For this review, use the dimensioned drawing (mm, ordinates from the lowest corner) and the shaded views. Round coordinates to 2 decimals unless told otherwise and drop trailing zeros. Write each loop counter-clockwise with the first axis right and the second up, starting at its lowest first coordinate (ties: lowest second). Pieces come first, ordered by that corner, then holes.
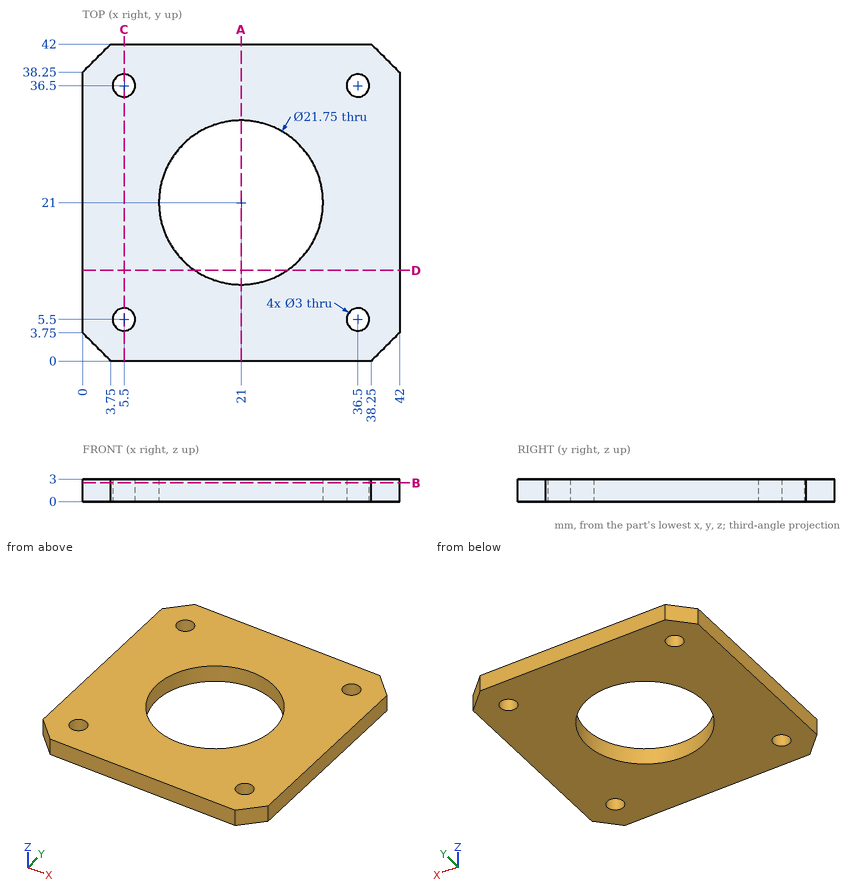
1) Add section B-B on z = 2.5. State the section outline as (x, y) points (3 decimals).
2) Add section A-A on x = 21. State the section outline as (y, z) points (3 decimals), and give its area (4 significant figures).
3) Add section D-D on y = 12. State the section outline as (x, z) points, and give its area (3 significant figures).
4) For line 1 along Y through (x, z) = (5.5, 1.1); line 2 along X through (y, z) = (36, 1.9); line 3 along X through (y, z) = (35.5, 1.95), list the stretches that pass through material, from the lowest coordinate up.
5) Add section C-C on x = 5.5. State the section outline as (y, z) points, and give its area (3 significant figures).
6) For P1, Ø2.5, axis at x = 5.5, y = 36.5, coming from the +Z side, flat-tipped, find the tip position at first contact; note if it passes through.
Computed:
1. outline: (0, 3.75) - (3.75, 0) - (38.25, 0) - (42, 3.75) - (42, 38.25) - (38.25, 42) - (3.75, 42) - (0, 38.25) - close; hole circle Ø3 at (5.5, 5.5); hole circle Ø3 at (5.5, 36.5); hole circle Ø21.75 at (21, 21); hole circle Ø3 at (36.5, 5.5); hole circle Ø3 at (36.5, 36.5)
2. outline: (0, 0) - (10.125, 0) - (10.125, 3) - (0, 3) - close; (31.875, 0) - (42, 0) - (42, 3) - (31.875, 3) - close
2. area: 60.75 mm2
3. outline: (0, 0) - (14.9, 0) - (14.9, 3) - (0, 3) - close; (27.1, 0) - (42, 0) - (42, 3) - (27.1, 3) - close
3. area: 89.4 mm2
4. line 1: y = 0 to 4, 7 to 35, 38 to 42
4. line 2: x = 0 to 4.09, 6.91 to 35.09, 37.91 to 42
4. line 3: x = 0 to 4.38, 6.62 to 35.38, 37.62 to 42
5. outline: (0, 0) - (4, 0) - (4, 3) - (0, 3) - close; (7, 0) - (35, 0) - (35, 3) - (7, 3) - close; (38, 0) - (42, 0) - (42, 3) - (38, 3) - close
5. area: 108 mm2
6. P1: passes through
